Design review of the part built by this model. Coordinates are the model's own, in mm. Face numbers are marked on the shaded views. A direction names the side the tool comes from. Round coordinates to 2 decimals unless told otherwise and drop trailing zeros. Loops run counter-clockwise (first coordinate to the right, second up) from the corner with the lowest first, then second, coordinate; pieces in that order, holes last. Notation, with made-up numbers: (11.25, 54) - (39.25, 54) arc R21 ccw to (39.25, 64) - close; hole circle Ø6 at (45, 51). An arc over 180 degrees is marked (long way). Use one line per item in the form item = value. Start each with the question number.
(1) The part is to be moulded in two halves that separate along Y. For the marked faces 1, 2, 3 and 4, say which applies: released by +Y, released by -Y, zero draft, split by the parting line, or undercut.
(2) Wall thickness on probe 1 along Z at (x, y) = (64, 13.5); probe 2 along Y at (x, z) = (41, 2); probe 3 along Z at (x, y) = (27.75, 20): over which ranges is each line inside the solid? List them lowest first. Write a range as [from, to].
(3) We need section A-A, the plane x = 5. Write out the cut boundary in (y, z).
(4) For pin 1 (1.5 mm diameter, centred on y = 99.5, z = 1.5, fed in from +X); pin 2 (8 mm diameter, centred on x = 67.5, y = 74, fed in from -Z); pin 3 (2 mm diameter, centred on x = 57, z = 10.5, fed in from +Y), all flat-tipped, find the tip position at first contact; note any pin that passes through.
(5) Machinability: for the marked faces 5, 6 and 7, which of the approach directions +Z, -Z, +X, -X, +Y, -Y give a long, thin tool a straight path to every point of the face, cutting with its end or side? Answer none if there is none.
(6) We need section C-C, the plane x = 53. Write out the cut boundary in (y, z), then the cut area to 3 significant figures.
(7) We need section B-B, the plane y = 54. Write out the cut boundary in (x, z).
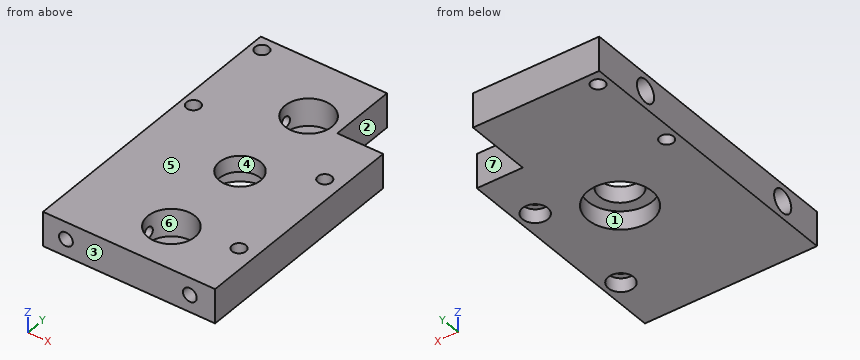
from build123d import *

# Parameters (mm, degrees)
F1_DEPTH  = 15
F2_R      = 3
F2_R_2    = 9
F3_DEPTH  = 15.001
F4_R      = 5.5
F5_DEPTH  = 6
F6_R      = 10.25
F7_DEPTH  = 12
F9_D      = 5
F9_DEPTH  = 35
F10_R     = 5
F10_R_2   = 2.5
F11_DEPTH = 18
F12_R     = 3
F13_DEPTH = 17.9
F14_R     = 14
F15_DEPTH = 8


with BuildPart() as f1:
    # F0 (on Top) → F1 (new body)
    with BuildSketch(Plane.XY):
        Polygon((0, 127), (0, 0), (75, 0), (75, 98), (55, 98), (55, 127), align=None)
    extrude(amount=F1_DEPTH)

    # F2 (on face) → F3 (cut, through all)
    with BuildSketch(Plane(origin=(0, 0, 0), x_dir=(1, 0, 0), z_dir=(0, 0, -1))):
        with Locations((5, -121)):
            Circle(F2_R)
        with Locations((5, -81)):
            Circle(F2_R)
        with Locations((41, -60)):
            Circle(F2_R_2)
        with Locations((67.5, -24)):
            Circle(F2_R)
        with Locations((67.5, -74)):
            Circle(F2_R)
    extrude(amount=-F3_DEPTH, mode=Mode.SUBTRACT)

    # F4 (on face) → F5 (cut)
    with BuildSketch(Plane(origin=(0, 0, 0), x_dir=(1, 0, 0), z_dir=(0, 0, -1))):
        with Locations((67.5, -74)):
            Circle(F4_R)
        with Locations((67.5, -24)):
            Circle(F4_R)
    extrude(amount=-F5_DEPTH, mode=Mode.SUBTRACT)

    # F6 (on face) → F7 (cut)
    with BuildSketch(Plane.XY.offset(15)):
        with Locations((41, 100)):
            Circle(F6_R)
        with Locations((41, 20)):
            Circle(F6_R)
    extrude(amount=-F7_DEPTH, mode=Mode.SUBTRACT)

    # F9
    with Locations(Plane(origin=(0, 0, 0), x_dir=(0, -1, 0), z_dir=(-1, 0, 0))):
        with Locations((-100, 7.5), (-20, 7.5)):
            Hole(F9_D / 2, depth=F9_DEPTH)

    # F10 (on face) → F11 (cut)
    with BuildSketch(Plane(origin=(0, 0, 0), x_dir=(0, -1, 0), z_dir=(-1, 0, 0))):
        with Locations((-100, 7.5)):
            Circle(F10_R)
        with Locations((-100, 7.5)):
            Circle(F10_R_2, mode=Mode.SUBTRACT)
        with Locations((-20, 7.5)):
            Circle(F10_R)
        with Locations((-20, 7.5)):
            Circle(F10_R_2, mode=Mode.SUBTRACT)
    extrude(amount=-F11_DEPTH, mode=Mode.SUBTRACT)

    # F12 (on face) → F13 (cut)
    with BuildSketch(Plane.XZ):
        with Locations((10, 7.5)):
            Circle(F12_R)
        with Locations((64, 7.5)):
            Circle(F12_R)
    extrude(amount=-F13_DEPTH, mode=Mode.SUBTRACT)

    # F14 (on face) → F15 (cut)
    with BuildSketch(Plane(origin=(0, 0, 0), x_dir=(1, 0, 0), z_dir=(0, 0, -1))):
        with Locations((41, -60)):
            Circle(F14_R)
    extrude(amount=-F15_DEPTH, mode=Mode.SUBTRACT)


solid = f1.part
Data:
q1.face_1 = undercut
q1.face_2 = zero draft
q1.face_3 = released by -Y
q1.face_4 = undercut
q2.probe_1 = [0, 4.5], [10.5, 15]
q2.probe_2 = [0, 46], [74, 127]
q2.probe_3 = [0, 5], [10, 15]
q3.outline = (0, 0) - (78, 0) - (78, 15) - (0, 15) - close; (84, 0) - (118, 0) - (118, 15) - (84, 15) - close; (124, 0) - (127, 0) - (127, 15) - (124, 15) - close; hole circle Ø10 at (20, 7.5); hole circle Ø10 at (100, 7.5)
q4.pin_1 = 55
q4.pin_2 = 6
q4.pin_3 = 98
q5.face_5 = +Z, +X, -X, +Y, -Y
q5.face_6 = +Z
q5.face_7 = +Z, -Z, +X, +Y
q6.outline = (0, 0) - (52.79, 0) - (52.79, 8) - (67.21, 8) - (67.21, 0) - (127, 0) - (127, 15) - (0, 15) - close
q6.area = 1,790 mm^2
q7.outline = (0, 0) - (28.35, 0) - (28.35, 8) - (34.29, 8) - (34.29, 15) - (0, 15) - close; (47.71, 8) - (53.65, 8) - (53.65, 0) - (75, 0) - (75, 15) - (47.71, 15) - close
